from build123d import *

# Parameters (mm, degrees)
SKETCH1_W                                  = 66.04
SKETCH1_H                                  = 73.66
BOSS_EXTRUDE1_DEPTH                        = 66.04
CONVERT_SOLID1_START                       = 10
CONVERT_SOLID1_OUTLINE_W                   = 66.04
CONVERT_SOLID1_OUTLINE_H                   = 73.66
CONVERT_SOLID1_DEPTH                       = 56.04
SKETCH12_W                                 = 61.174671733
SKETCH12_H                                 = 67.796672281
CUT_EXTRUDE1_DEPTH                         = 71.66800329
FILLET1_R                                  = 2.54
CBORE_FOR_8_FILLISTER_HEAD_MACHINE_2_COUNT = 2
CBORE_FOR_8_FILLISTER_HEAD_MACHINE_2_PITCH = 48.289098212
LPATTERN1_COUNT                            = 2
LPATTERN1_PITCH                            = 63.5


# Read off the part's stored shape, not the designer's step: Convert-Solid1
with BuildPart() as part:
    # Sketch1 → Boss-Extrude1 (new body)
    with BuildSketch(Plane.XY):
        with Locations((-6.510518448, 20.887456633)):
            Rectangle(SKETCH1_W, SKETCH1_H)
    extrude(amount=BOSS_EXTRUDE1_DEPTH)

    # Convert-Solid1 outline → Convert-Solid1 (cut)
    with BuildSketch(Plane.XY.offset(CONVERT_SOLID1_START)):
        with Locations((-6.510518448, 20.887456633)):
            Rectangle(CONVERT_SOLID1_OUTLINE_W, CONVERT_SOLID1_OUTLINE_H)
    extrude(amount=CONVERT_SOLID1_DEPTH, mode=Mode.SUBTRACT)

    # Sketch12 → Cut-Extrude1 (cut, symmetric)
    with BuildSketch(Plane(origin=(0, 0, 0), x_dir=(-1, 0, 0), z_dir=(0, 0, -1))):
        with Locations((6.563074008, 21.518123352)):
            Rectangle(SKETCH12_W, SKETCH12_H)
    cut_extrude1 = extrude(amount=CUT_EXTRUDE1_DEPTH, both=True, mode=Mode.SUBTRACT)

    # Fillet1
    fillet1_edges = [part.edges().sort_by_distance(p)[0] for p in [
        (-39.530518448, 57.717456633, 5),
        (-39.530518448, -15.942543367, 5),
        (26.509481552, -15.942543367, 5),
        (26.509481552, 57.717456633, 5),
    ]]
    fillet(fillet1_edges, radius=FILLET1_R)

    # Sketch18 → CBORE for #8 Fillister Head Machine Screw1 (revolve, cut)
    with BuildSketch(Plane(origin=(26.509481552, 46.108209089, 5.16610426), x_dir=(0, 0, -1), z_dir=(0, 1, 0))):
        Polygon((0, 0), (0, 26.750674586), (2.2479, 25.4), (2.2479, 3.9624), (3.77063, 3.9624), (3.77063, 0.635), (4.40563, 0), align=None)
    cbore_for_8_fillister_head_machine_scre = revolve(axis=Axis((32.859481552, 46.108209089, 5.16610426), (-1, 0, 0)), mode=Mode.SUBTRACT)

    # CBORE for _8 Fillister Head Machine  2: CBORE for #8 Fillister Head Machine Screw1 ×2
    with Locations(*[Vector(0, -0.9998317064949376, -0.018345535898989723) * (i * CBORE_FOR_8_FILLISTER_HEAD_MACHINE_2_PITCH) for i in range(1, CBORE_FOR_8_FILLISTER_HEAD_MACHINE_2_COUNT)]):
        add(cbore_for_8_fillister_head_machine_scre, mode=Mode.SUBTRACT)

    # LPattern1: Cut-Extrude1, CBORE for #8 Fillister Head Machine Screw1 ×2
    with Locations(*[(-i * LPATTERN1_PITCH, 0, 0) for i in range(1, LPATTERN1_COUNT)]):
        add(cut_extrude1, mode=Mode.SUBTRACT)
        add(cbore_for_8_fillister_head_machine_scre, mode=Mode.SUBTRACT)

    # LPattern1 copy 1 sketch → LPattern1 copy 1 (revolve, cut)
    with BuildSketch(Plane(origin=(-36.990518448, -2.172762381, 4.280214875), x_dir=(0, 0, -1), z_dir=(0, 1, 0))):
        Polygon((0, 0), (0, 26.750674586), (2.2479, 25.4), (2.2479, 3.9624), (3.77063, 3.9624), (3.77063, 0.635), (4.40563, 0), align=None)
    revolve(axis=Axis((-30.640518448, -2.172762381, 4.280214875), (-1, 0, 0)), mode=Mode.SUBTRACT)


solid = part.part
The listing builds one solid part. Answer for the finished solid, in the listing's coordinates (mm). A direction names the side the tool comes from. Round coordinates to 2 decimals unless told otherwise and drop trailing zeros. Write each loop counter-clockwise with the first axis right and the second up, starting at its lowest first coordinate (ties: lowest second). Pieces come first, ordered by that corner, then holes. Notation, with made-up numbers: (73, 86) - (92, 86) arc R16 ccw to (92, 90) - close; hole circle Ø10 at (-35, 67). An arc over 180 degrees is marked (long way). Use a Markdown table: item, result. Add a question column.
1. Consider line 1 (X direction, y = -2, z = 9.5); line 2 (Y direction, x = -4, z = 2); line 3 (X direction, y = 2, z = 4.75). Determine where each line is inside the solid, lowest interval first.
2. The part is cut by section A-A (x = 9.5). Write down the section's boundary in (y, z).
3. The part is cut by section B-B (y = 31). Write down the section's boundary in (x, z).
4. For a pull along Y with two mould halves and no side action, classify faces 1 (the face through (-7, 57.717, 5)), 2 (the face through (-38.538, -3.305, 0.684)), 3 (the face through (-38.806, -15.179, 5.07)) as +Y half, -Y half, draft (parallel to the pull), parting line (faces both ways), or undercut.
5. A flat-ended cylindrical pin translates along its axis: P1, Ø4.5, axis at y = 46.11, z = 5.17, coming from the -X side. Find the tip coordinate at first contact, or state that the pin passes through.
6. The part is cut by section C-C (z = 5.25). Give the number of separate pieces and of enclosed holes in the cut face, and give its area (3 significant figures).
7. A tool of negligible diameter and unlimited length cuts with its end or side. For faces 4 (the face through (-7, -15.943, 5)), 5 (the face through (-37.15, 21, 5)), from which of +Z, -Z, +X, -X, +Y, -Y can it reach the whole face along a straight path? Write none if from no direction.
Reported:
| question | item | result |
|---|---|---|
| 1 | line 1 | -39.48 to -37.15, 24.02 to 26.51 |
| 1 | line 2 | -15.94 to -12.38, 55.42 to 57.72 |
| 1 | line 3 | -39.48 to -37.2, 24.02 to 26.3 |
| 2 | outline | (-15.94, 0) - (-12.38, 0) - (-12.38, 10) - (-15.94, 10) - close; (55.42, 0) - (57.72, 0) - (57.72, 10) - (55.42, 10) - close |
| 3 | outline | (-39.48, 0) - (-37.15, 0) - (-37.15, 10) - (-39.48, 10) - close; (24.02, 0) - (26.51, 0) - (26.51, 10) - (24.02, 10) - close |
| 4 | face 1 | +Y half |
| 4 | face 2 | undercut |
| 4 | face 3 | -Y half |
| 5 | P1 | through |
| 6 | separate pieces | 4 |
| 6 | enclosed holes | 0 |
| 6 | area | 635 mm^2 |
| 7 | face 4 | +Z, -Z, +X, -X, -Y |
| 7 | face 5 | +Z, -Z |
